Source: CAD feature listing. Evaluate the final solid. Frame: model axes, mm. Coordinates: 2 decimals unless noted, no trailing zeros. Write each loop counter-clockwise with the first axis right and the second up, starting at its lowest first coordinate (ties: lowest second). Pieces come first, ordered by that corner, then holes. Notation, with made-up numbers: (-38.75, -9.5) -> (-9.75, -9.5) arc R9 ccw to (-9.75, 2.5) -> close; hole circle Ø5 at (20, -18). An arc over 180 degrees is marked (long way). One line per item, written item: value. Start each with the question number.
1. Section query A-A, the plane x = 0. Output: boundary loops of the cut face in (y, z), and give its area (3 significant figures).
2. Line query: line 1 (X direction, y = 60.5, z = 0.3); line 2 (Y direction, x = 37.5, z = 0.7); line 3 (X direction, y = 60, z = 1.4). Output: solid intervals per line, ascending.
3. First-contact query: P1, Ø1.5, axis at y = -64.5, z = 3, coming from the +X side; P2, Ø1, axis at x = 26.5, z = 1.5, coming from the -Y side; P3, Ø1.5, axis at x = -61, z = 3.5, coming from the -Y side. Flat tips, straight axial feed; report the tip coordinate or a pass-through.
4. Section query D-D, the plane x = -26.5. Output: boundary loops of the cut face in (y, z).
5. Section query C-C, the plane x = 60. Output: boundary loops of the cut face in (y, z).
from build123d import *

# Parameters (mm, degrees)
F0_R     = 6.35
F1_DEPTH = 5.08


with BuildPart() as f1:
    # F0 (on Top) → F1 (new body)
    with BuildSketch(Plane.XY):
        with BuildLine():
            Line((-4.392071, 67.140981), (-4.392071, 56.980981))
            ThreePointArc((-4.392071, 56.980981), (-8.94023, 56.446389), (-13.430984, 55.549358))
            Line((-13.430984, 55.549358), (-16.570597, 65.212092))
            ThreePointArc((-16.570597, 65.212092), (-21.253073, 65.410232), (-24.924812, 62.497643))
            Line((-24.924812, 62.497643), (-21.785199, 52.834909))
            ThreePointArc((-21.785199, 52.834909), (-25.945557, 50.921023), (-29.939321, 48.680176))
            Line((-29.939321, 48.680176), (-35.911219, 56.899789))
            ThreePointArc((-35.911219, 56.899789), (-40.425746, 55.641266), (-43.017738, 51.7366))
            Line((-43.017738, 51.7366), (-37.04584, 43.516988))
            ThreePointArc((-37.04584, 43.516988), (-40.411153, 40.411153), (-43.516988, 37.04584))
            Line((-43.516988, 37.04584), (-51.7366, 43.017738))
            ThreePointArc((-51.7366, 43.017738), (-55.641266, 40.425746), (-56.899789, 35.911219))
            Line((-56.899789, 35.911219), (-48.680176, 29.939321))
            ThreePointArc((-48.680176, 29.939321), (-50.921023, 25.945557), (-52.834909, 21.785199))
            Line((-52.834909, 21.785199), (-62.497643, 24.924812))
            ThreePointArc((-62.497643, 24.924812), (-65.410232, 21.253073), (-65.212092, 16.570597))
            Line((-65.212092, 16.570597), (-55.549358, 13.430984))
            ThreePointArc((-55.549358, 13.430984), (-56.446389, 8.94023), (-56.980981, 4.392071))
            Line((-56.980981, 4.392071), (-67.140981, 4.392071))
            ThreePointArc((-67.140981, 4.392071), (-68.776388, 0), (-67.140981, -4.392071))
            Line((-67.140981, -4.392071), (-56.980981, -4.392071))
            ThreePointArc((-56.980981, -4.392071), (-56.446389, -8.94023), (-55.549358, -13.430984))
            Line((-55.549358, -13.430984), (-65.212092, -16.570597))
            ThreePointArc((-65.212092, -16.570597), (-65.410232, -21.253073), (-62.497643, -24.924812))
            Line((-62.497643, -24.924812), (-52.834909, -21.785199))
            ThreePointArc((-52.834909, -21.785199), (-50.921023, -25.945557), (-48.680176, -29.939321))
            Line((-48.680176, -29.939321), (-56.899789, -35.911219))
            ThreePointArc((-56.899789, -35.911219), (-55.641266, -40.425746), (-51.7366, -43.017738))
            Line((-51.7366, -43.017738), (-43.516988, -37.04584))
            ThreePointArc((-43.516988, -37.04584), (-40.411153, -40.411153), (-37.04584, -43.516988))
            Line((-37.04584, -43.516988), (-43.017738, -51.7366))
            ThreePointArc((-43.017738, -51.7366), (-40.425746, -55.641266), (-35.911219, -56.899789))
            Line((-35.911219, -56.899789), (-29.939321, -48.680176))
            ThreePointArc((-29.939321, -48.680176), (-25.945557, -50.921023), (-21.785199, -52.834909))
            Line((-21.785199, -52.834909), (-24.924812, -62.497643))
            ThreePointArc((-24.924812, -62.497643), (-21.253073, -65.410232), (-16.570597, -65.212092))
            Line((-16.570597, -65.212092), (-13.430984, -55.549358))
            ThreePointArc((-13.430984, -55.549358), (-8.94023, -56.446389), (-4.392071, -56.980981))
            Line((-4.392071, -56.980981), (-4.392071, -67.140981))
            ThreePointArc((-4.392071, -67.140981), (0, -68.776388), (4.392071, -67.140981))
            Line((4.392071, -67.140981), (4.392071, -56.980981))
            ThreePointArc((4.392071, -56.980981), (8.94023, -56.446389), (13.430984, -55.549358))
            Line((13.430984, -55.549358), (16.570597, -65.212092))
            ThreePointArc((16.570597, -65.212092), (21.253073, -65.410232), (24.924812, -62.497643))
            Line((24.924812, -62.497643), (21.785199, -52.834909))
            ThreePointArc((21.785199, -52.834909), (25.945557, -50.921023), (29.939321, -48.680176))
            Line((29.939321, -48.680176), (35.911219, -56.899789))
            ThreePointArc((35.911219, -56.899789), (40.425746, -55.641266), (43.017738, -51.7366))
            Line((43.017738, -51.7366), (37.04584, -43.516988))
            ThreePointArc((37.04584, -43.516988), (40.411153, -40.411153), (43.516988, -37.04584))
            Line((43.516988, -37.04584), (51.7366, -43.017738))
            ThreePointArc((51.7366, -43.017738), (55.641266, -40.425746), (56.899789, -35.911219))
            Line((56.899789, -35.911219), (48.680176, -29.939321))
            ThreePointArc((48.680176, -29.939321), (50.921023, -25.945557), (52.834909, -21.785199))
            Line((52.834909, -21.785199), (62.497643, -24.924812))
            ThreePointArc((62.497643, -24.924812), (65.410232, -21.253073), (65.212092, -16.570597))
            Line((65.212092, -16.570597), (55.549358, -13.430984))
            ThreePointArc((55.549358, -13.430984), (56.446389, -8.94023), (56.980981, -4.392071))
            Line((56.980981, -4.392071), (67.140981, -4.392071))
            ThreePointArc((67.140981, -4.392071), (68.776388, 0), (67.140981, 4.392071))
            Line((67.140981, 4.392071), (56.980981, 4.392071))
            ThreePointArc((56.980981, 4.392071), (56.446389, 8.94023), (55.549358, 13.430984))
            Line((55.549358, 13.430984), (65.212092, 16.570597))
            ThreePointArc((65.212092, 16.570597), (65.410232, 21.253073), (62.497643, 24.924812))
            Line((62.497643, 24.924812), (52.834909, 21.785199))
            ThreePointArc((52.834909, 21.785199), (50.921023, 25.945557), (48.680176, 29.939321))
            Line((48.680176, 29.939321), (56.899789, 35.911219))
            ThreePointArc((56.899789, 35.911219), (55.641266, 40.425746), (51.7366, 43.017738))
            Line((51.7366, 43.017738), (43.516988, 37.04584))
            ThreePointArc((43.516988, 37.04584), (40.411153, 40.411153), (37.04584, 43.516988))
            Line((37.04584, 43.516988), (43.017738, 51.7366))
            ThreePointArc((43.017738, 51.7366), (40.425746, 55.641266), (35.911219, 56.899789))
            Line((35.911219, 56.899789), (29.939321, 48.680176))
            ThreePointArc((29.939321, 48.680176), (25.945557, 50.921023), (21.785199, 52.834909))
            Line((21.785199, 52.834909), (24.924812, 62.497643))
            ThreePointArc((24.924812, 62.497643), (21.253073, 65.410232), (16.570597, 65.212092))
            Line((16.570597, 65.212092), (13.430984, 55.549358))
            ThreePointArc((13.430984, 55.549358), (8.94023, 56.446389), (4.392071, 56.980981))
            Line((4.392071, 56.980981), (4.392071, 67.140981))
            ThreePointArc((4.392071, 67.140981), (0, 68.776388), (-4.392071, 67.140981))
        make_face()
        Circle(F0_R, mode=Mode.SUBTRACT)
    extrude(amount=F1_DEPTH)


solid = f1.part
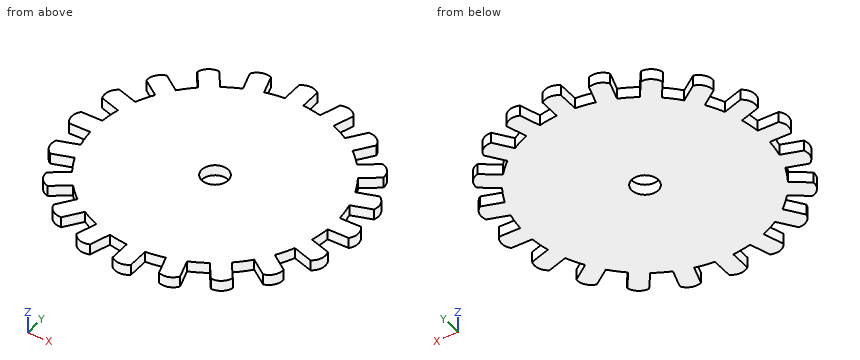
Computed values:
1. outline: (-68.78, 0) -> (-6.35, 0) -> (-6.35, 5.08) -> (-68.78, 5.08) -> close; (6.35, 0) -> (68.78, 0) -> (68.78, 5.08) -> (6.35, 5.08) -> close
1. area: 634 mm²
2. line 1: x = -24.28 to -15.04, -4.39 to 4.39, 15.04 to 24.28
2. line 2: y = -56.85 to -44.14, -43.13 to 43.13, 44.14 to 56.85
2. line 3: x = -24.11 to -14.88, -4.39 to 4.39, 14.88 to 24.11
3. P1: stops at x = 23.95
3. P2: stops at y = -50.89
3. P3: stops at y = -24.68
4. outline: (-50.63, 0) -> (50.63, 0) -> (50.63, 5.08) -> (-50.63, 5.08) -> close
5. outline: (-24.11, 0) -> (-14.88, 0) -> (-14.88, 5.08) -> (-24.11, 5.08) -> close; (-4.39, 0) -> (4.39, 0) -> (4.39, 5.08) -> (-4.39, 5.08) -> close; (14.88, 0) -> (24.11, 0) -> (24.11, 5.08) -> (14.88, 5.08) -> close
